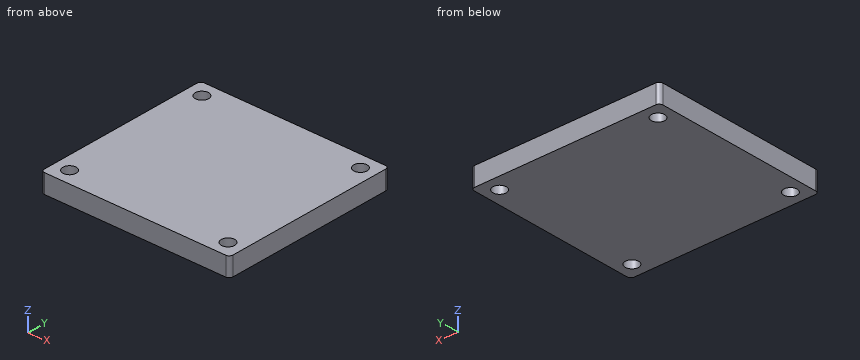
from build123d import *

# Parameters (mm, degrees)
SKETCH1_W             = 63.5
SKETCH1_H             = 59.69
BOSS_EXTRUDE1_DEPTH   = 6.35
FILLET1_R             = 1.27
F_8_CLEARANCE_HOLE1_D = 4.4958


with BuildPart() as part:
    # Sketch1 → Boss-Extrude1 (new body)
    with BuildSketch(Plane.XY):
        with Locations((31.75, 29.845)):
            Rectangle(SKETCH1_W, SKETCH1_H)
    extrude(amount=BOSS_EXTRUDE1_DEPTH)

    # Fillet1
    fillet1_edges = [part.edges().sort_by_distance(p)[0] for p in [
        (0, 59.69, 3.175),
        (63.5, 59.69, 3.175),
        (63.5, 0, 3.175),
        (0, 0, 3.175),
    ]]
    fillet(fillet1_edges, radius=FILLET1_R)

    # #8 Clearance Hole1 (through all)
    with Locations(Plane.XY.offset(6.35)):
        with Locations((5.08, 54.61), (58.42, 54.61), (58.42, 5.08), (5.08, 5.08)):
            Hole(F_8_CLEARANCE_HOLE1_D / 2)


solid = part.part
CAD build for the part. Positions are in the model's coordinates, mm. Give positions to 0.01 mm unless a question says otherwise; leave off trailing zeros. Loops run counter-clockwise (first coordinate to the right, second up) from the corner with the lowest first, then second, coordinate; pieces in that order, holes last. Notation, with made-up numbers: M -17.75,36.25 L 4.25,36.25 A22 cw 4.25,56.25 Z; hole C -34.75,9.5 d9. An arc over 180 degrees is marked long. Answer in a Markdown table with one row per item. Add a question column.
Item 1: Band-saw the part on A-A on x = 5.08. Give the cut face in (y, z).
Item 2: Band-saw the part on B-B on y = 54.61. Give the cut face in (x, z), then the cut area to 3 significant figures.
Item 3: Band-saw the part on C-C on z = 2.75. Give the cut face in (x, y).
Item 4: Probe probe 1 along Y at (x, z) = (58.42, 2.5); probe 2 along X at (y, z) = (6.5, 2.75); probe 3 along Y at (x, z) = (57, 5.5). List the from-to ranges inside material, lowest first.
Reply:
| question | item | result |
|---|---|---|
| 1 | outline | M 0,0 L 2.83,0 L 2.83,6.35 L 0,6.35 Z; M 7.33,0 L 52.36,0 L 52.36,6.35 L 7.33,6.35 Z; M 56.86,0 L 59.69,0 L 59.69,6.35 L 56.86,6.35 Z |
| 2 | outline | M 0,0 L 2.83,0 L 2.83,6.35 L 0,6.35 Z; M 7.33,0 L 56.17,0 L 56.17,6.35 L 7.33,6.35 Z; M 60.67,0 L 63.5,0 L 63.5,6.35 L 60.67,6.35 Z |
| 2 | area | 346 mm^2 |
| 3 | outline | M 0,1.27 A1.27 ccw 1.27,0 L 62.23,0 A1.27 ccw 63.5,1.27 L 63.5,58.42 A1.27 ccw 62.23,59.69 L 1.27,59.69 A1.27 ccw 0,58.42 Z; hole C 5.08,5.08 d4.5; hole C 5.08,54.61 d4.5; hole C 58.42,5.08 d4.5; hole C 58.42,54.61 d4.5 |
| 4 | probe 1 | y = 0 to 2.83, 7.33 to 52.36, 56.86 to 59.69 |
| 4 | probe 2 | x = 0 to 3.34, 6.82 to 56.68, 60.16 to 63.5 |
| 4 | probe 3 | y = 0 to 3.34, 6.82 to 52.87, 56.35 to 59.69 |
